For this review, take the finished solid that the model builds, in its own axes (mm). Round coordinates to 2 decimals unless told otherwise and drop trailing zeros. Order: outer loops, then holes, each group sorted by start corner. A loop starts at its lowest first (then second) coordinate and runs counter-clockwise, first axis right, second up. Notation, with made-up numbers: M -33.5,59 L 5.5,59 A29 cw 5.5,89 Z; hole C -18.75,48.25 d1. An arc over 180 degrees is marked long. Use a Markdown table: item, result.
from build123d import *

# Parameters (mm, degrees)
F0_W     = 457.2
F0_H     = 609.6
F1_DEPTH = 25.4
F2_R     = 6.35
F3_DEPTH = 762
F4_R     = 6.35
F5_DEPTH = 25.4


with BuildPart() as f1:
    # F0 (on Top) → F1 (new body)
    with BuildSketch(Plane.XY):
        Rectangle(F0_W, F0_H)
    extrude(amount=F1_DEPTH)

    # F2 (on face) → F3 (cut)
    with BuildSketch(Plane.YZ.offset(228.6)):
        with Locations((0, 12.7)):
            Circle(F2_R)
    extrude(amount=-F3_DEPTH, mode=Mode.SUBTRACT)

    # F4 (on face) → F5 (cut)
    with BuildSketch(Plane.XY.offset(25.4)):
        Circle(F4_R)
    extrude(amount=-F5_DEPTH, mode=Mode.SUBTRACT)


solid = f1.part
Q1. Wall thickness on line 1 along Z through (x, y) = (173, 0); line 2 along Y through (x, z) = (0, 8); line 3 along X through (y, z) = (0, 6): over which ranges is each line inside the solid? List them lowest first. Write a range as [from, to].
Determined:
| item | result |
|---|---|
| line 1 | z = [0, 6.35], [19.05, 25.4] |
| line 2 | y = [-304.8, -6.35], [6.35, 304.8] |
| line 3 | x = [-228.6, -6.35], [6.35, 228.6] |
Q2. Draft analysis for pull direction X (two halves, no side actions). For faces 1 (the flat face through (48, 4, 0)), 2 (the flat face through (-228.6, -4, 18)), 3 (the cylindrical face through (3.414, 5.354, 20.55)), state which applies: pulls with the +X half, pulls with the -X half, needs draft (parallel to the pull), parting line crosses it, or undercut.
Determined:
| item | result |
|---|---|
| face 1 | needs draft |
| face 2 | pulls with the -X half |
| face 3 | undercut |
Q3. Add section A-A (y = 0). Write out the cut boundary in (x, z), then the cut area to 3 significant figures.
Determined:
| item | result |
|---|---|
| outline | M -228.6,0 L -6.35,0 L -6.35,6.35 L -228.6,6.35 Z; M -228.6,19.05 L -6.35,19.05 L -6.35,25.4 L -228.6,25.4 Z; M 6.35,0 L 228.6,0 L 228.6,6.35 L 6.35,6.35 Z; M 6.35,19.05 L 228.6,19.05 L 228.6,25.4 L 6.35,25.4 Z |
| area | 5,650 mm^2 |
